Build history of the part. All positions in model axes, mm. Face numbers are marked on the shaded views. A direction names the side the tool comes from. Round coordinates to 2 decimals unless told otherwise and drop trailing zeros. Loops run counter-clockwise (first coordinate to the right, second up) from the corner with the lowest first, then second, coordinate; pieces in that order, holes last.
from build123d import *

# Parameters (mm, degrees)
BOSS_EXTRU_1_DEPTH      = 5
ESQUISSE2_R             = 3.5
ENL_V_MAT_EXTRU_1_DEPTH = 5
BOSS_EXTRU_2_DEPTH      = 5
BOSS_EXTRU_2_DEPTH_BACK = 10
ESQUISSE3_W             = 20
ESQUISSE3_H             = 3
ESQUISSE4_R             = 1
ENL_V_MAT_EXTRU_2_DEPTH = 5


with BuildPart() as part:
    # Esquisse1 → Boss.-Extru.1 (new body)
    with BuildSketch(Plane.XY):
        with BuildLine():
            Line((-10, -28.63), (-10, 0))
            ThreePointArc((-10, 0), (0, 10), (10, 0))
            Line((10, 0), (10, -28.63))
            Line((10, -28.63), (-10, -28.63))
        make_face()
    extrude(amount=BOSS_EXTRU_1_DEPTH)

    # Esquisse2 → Enlèv. mat.-Extru.1 (cut)
    with BuildSketch(Plane.XY.offset(5)):
        Circle(ESQUISSE2_R)
    extrude(amount=-ENL_V_MAT_EXTRU_1_DEPTH, mode=Mode.SUBTRACT)

    # Esquisse3 → Boss.-Extru.2 (add, two sides: drawn at the far end of the back side and taken through both)
    with BuildSketch(Plane.XY.offset(5).offset(-BOSS_EXTRU_2_DEPTH_BACK)):
        with Locations((0, -27.13)):
            Rectangle(ESQUISSE3_W, ESQUISSE3_H)
    extrude(amount=BOSS_EXTRU_2_DEPTH + BOSS_EXTRU_2_DEPTH_BACK)

    # Esquisse4 → Enlèv. mat.-Extru.2 (cut)
    with BuildSketch(Plane(origin=(0, -25.63, 0), x_dir=(1, 0, 0), z_dir=(0, 1, 0))):
        with Locations(Location((-7, -7.92068908, 0), (0, 0, 270))):
            Circle(ESQUISSE4_R)
        with Locations(Location((7.865355749, -7.92068908, 0), (0, 0, 270))):
            Circle(ESQUISSE4_R)
        with Locations(Location((7.865355749, 2.5, 0), (0, 0, 270))):
            Circle(ESQUISSE4_R)
        with Locations(Location((-7, 2.5, 0), (0, 0, 270))):
            Circle(ESQUISSE4_R)
    extrude(amount=-ENL_V_MAT_EXTRU_2_DEPTH, mode=Mode.SUBTRACT)


solid = part.part
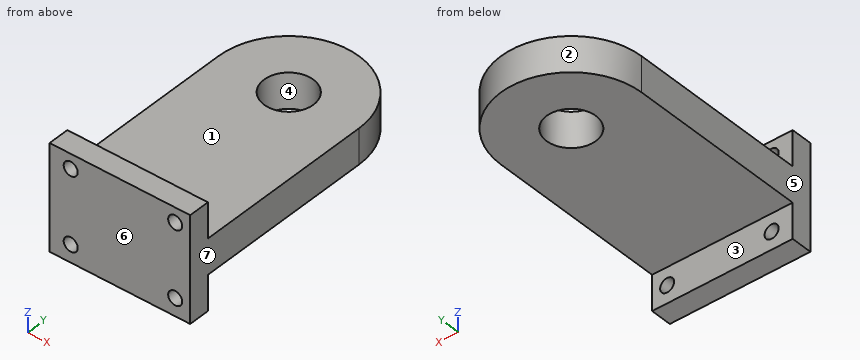
(1) Slice it at A-A on z = -2.5. List the corners of the cut face in (x, y).
Responses:
outline: (-10, -28.63) - (-8, -28.63) - (-8, -25.63) - (-10, -25.63) - close; (-6, -28.63) - (6.87, -28.63) - (6.87, -25.63) - (-6, -25.63) - close; (8.87, -28.63) - (10, -28.63) - (10, -25.63) - (8.87, -25.63) - close
(2) Pin check, flat tips, straight feed: P1, Ø6, axis at x = -1, y = -6, coming from the +Z side; P2, Ø8, axis at x = -5, z = 1.5, coming from the +Y side; P3, Ø2.5, axis at x = 7.87, z = -2.5, coming from the +Y side. Stop position of each tip, or through.
Responses:
P1: stops at z = 5
P2: stops at y = 9.95
P3: stops at y = -25.63
(3) Which spindle directions (+Z, -Z, +X, -X, +Y, -Y) get a long thin tool onto all of the face, cutting with end or side? Do the marked faces 1, 2 and 3. Say none if no direction does.
Responses:
face 1: +Z, +X, -X, +Y
face 2: +Z, -Z, +Y
face 3: -Z, +X, -X, +Y
(4) Slice it at B-B on x = 0. List the corners of the cut face in (y, z), plus the area to 3 significant figures.
Responses:
outline: (-28.63, -5) - (-25.63, -5) - (-25.63, 0) - (-3.5, 0) - (-3.5, 5) - (-25.63, 5) - (-25.63, 10) - (-28.63, 10) - close; (3.5, 0) - (10, 0) - (10, 5) - (3.5, 5) - close
area: 188 mm2
(5) Pull direction X, two halves, no side cores. Call the marked faces 4, 5, 6 and 7: +X half, -X half, draft (parallel to the pull), parting line (faces both ways), or undercut.
Responses:
face 4: undercut
face 5: -X half
face 6: draft
face 7: +X half
(6) Probe line 1 (X direction, y = -27.55, z = -2.5); line 2 (Z direction, x = -0.75, y = -23); line 3 (Y direction, x = 1, z = 7.75). List the from-to ranges inside material, lowest first.
Responses:
line 1: x = -10 to -8, -6 to 6.87, 8.87 to 10
line 2: z = 0 to 5
line 3: y = -28.63 to -25.63
(7) Slice it at C-C on z = 3.5. List the corners of the cut face in (x, y).
Responses:
outline: (-10, -28.63) - (10, -28.63) - (10, 0) arc R10 ccw to (-10, 0) - close; hole circle Ø7 at (0, 0)
(8) Slice it at D-D on x = -7. List the corners of the cut face in (y, z), plus the area to 3 significant figures.
Responses:
outline: (-28.63, -5) - (-25.63, -5) - (-25.63, -3.5) - (-28.63, -3.5) - close; (-28.63, -1.5) - (-25.63, -1.5) - (-25.63, 0) - (7.14, 0) - (7.14, 5) - (-25.63, 5) - (-25.63, 6.92) - (-28.63, 6.92) - close; (-28.63, 8.92) - (-25.63, 8.92) - (-25.63, 10) - (-28.63, 10) - close
area: 197 mm2
